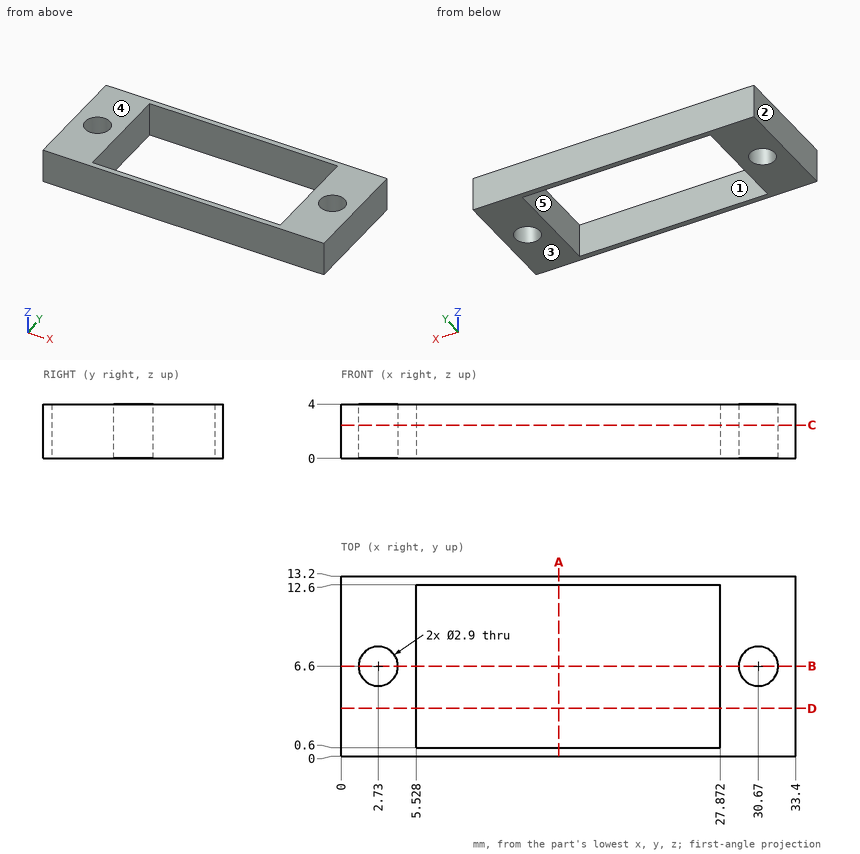
For this review, use the dimensioned drawing (mm, ordinates from the lowest corner) and the shaded views. A direction names the side the tool comes from. Coordinates: 2 decimals unless noted, no trailing zeros. Order: outer loops, then holes, each group sorted by start corner. A loop starts at its lowest first (then second) coordinate and runs counter-clockwise, first axis right, second up. Notation, with made-up numbers: (35.25, -4.75) - (67.25, -4.75) arc R17 ccw to (67.25, 13.25) - close; hole circle Ø5 at (41, -23). An arc over 180 degrees is marked (long way). Answer in a Markdown table with one row per item.
(1) Consider section C-C on z = 2.45. State the section outline as (x, y) points.
Checked values:
| item | result |
|---|---|
| outline | (0, 0) - (33.4, 0) - (33.4, 13.2) - (0, 13.2) - close; hole circle Ø2.9 at (2.73, 6.6); hole (5.53, 0.6) - (27.87, 0.6) - (27.87, 12.6) - (5.53, 12.6) - close; hole circle Ø2.9 at (30.67, 6.6) |
(2) Consider section A-A on x = 16. State the section outline as (y, z) points.
Checked values:
| item | result |
|---|---|
| outline | (0, 0) - (0.6, 0) - (0.6, 4) - (0, 4) - close; (12.6, 0) - (13.2, 0) - (13.2, 4) - (12.6, 4) - close |
(3) Consider section D-D on y = 3.5. State the section outline as (x, z) points.
Checked values:
| item | result |
|---|---|
| outline | (0, 0) - (5.53, 0) - (5.53, 4) - (0, 4) - close; (27.87, 0) - (33.4, 0) - (33.4, 4) - (27.87, 4) - close |
(4) For the marked faces 4 and 5, list the 3-axis set-ups (+Z, -Z, +X, -X, +Y, -Y) from which the entire face can be reached by the end or side of a thin tool; tool diameter is ignored.
Checked values:
| item | result |
|---|---|
| face 4 | +Z, +X, -X, +Y, -Y |
| face 5 | +Z, -Z |
(5) Consider section B-B on y = 6.6. State the section outline as (x, z) points.
Checked values:
| item | result |
|---|---|
| outline | (0, 0) - (1.28, 0) - (1.28, 4) - (0, 4) - close; (4.18, 0) - (5.53, 0) - (5.53, 4) - (4.18, 4) - close; (27.87, 0) - (29.22, 0) - (29.22, 4) - (27.87, 4) - close; (32.12, 0) - (33.4, 0) - (33.4, 4) - (32.12, 4) - close |
(6) The part is to be moulded in two halves that separate along X. For the marked faces 1, 2 and 3, say which applies: released by +X, released by -X, zero draft, split by the parting line, or undercut.
Checked values:
| item | result |
|---|---|
| face 1 | undercut |
| face 2 | released by -X |
| face 3 | zero draft |
(7) Wall thickness on line 1 along Y through (x, z) = (17, 2.85); line 2 along Y through (x, z) = (30.67, 3.1); line 3 along X through (y, z) = (9.75, 0.35): over which ranges is each line inside the solid? List them lowest first. Write a range as from..to.
Checked values:
| item | result |
|---|---|
| line 1 | 0..0.6, 12.6..13.2 |
| line 2 | 0..5.15, 8.05..13.2 |
| line 3 | 0..5.53, 27.87..33.4 |
